from build123d import *

# Parameters (mm, degrees)
F1_DEPTH = 63.5
F2_DEPTH = 63.5


with BuildPart() as f1:
    # F0 (on Top) → F1 (new body)
    with BuildSketch(Plane.XY):
        Polygon((61.167741, 31.75), (-65.832259, 31.75), (-65.58761, 0), (-2.332259, 0), (-2.332259, 12.7), (15.4492, 12.7), (61.167741, 12.7), align=None)
    extrude(amount=F1_DEPTH)

    # F0 (on Top) → F2 (join)
    with BuildSketch(Plane.XY):
        Polygon((61.167741, 31.75), (-65.832259, 31.75), (-65.58761, 0), (-2.332259, 0), (-2.332259, 12.7), (15.4492, 12.7), (61.167741, 12.7), align=None)
    extrude(amount=F2_DEPTH)


solid = f1.part
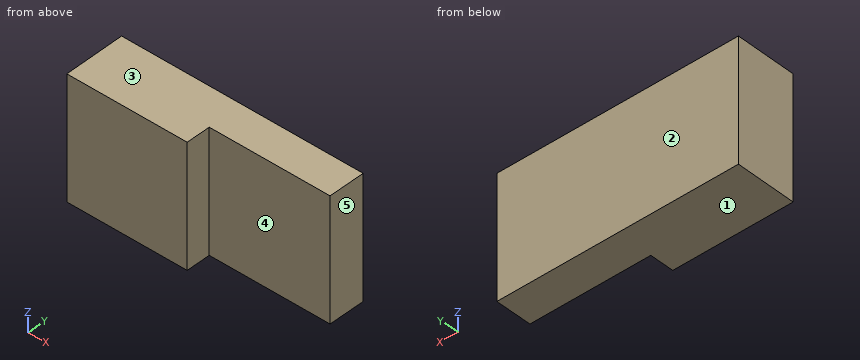
CAD build for the part. Positions are in the model's coordinates, mm. Face numbers are marked on the shaded views. A direction names the side the tool comes from. Coordinates: 2 decimals unless noted, no trailing zeros. Loops run counter-clockwise (first coordinate to the right, second up) from the corner with the lowest first, then second, coordinate; pieces in that order, holes last. Notation, with made-up numbers: (42, 78) - (46, 78) arc R20 cw to (46, 102) - close; hole circle Ø4 at (55, -21.5). An arc over 180 degrees is marked (long way). Use one line per item in the form item = value. Start each with the question number.
1) Band-saw the part on C-C (y = 6.5). Give the cut face in (x, z), and give its area (3 significant figures).
2) Tool access for the marked faces 4 and 5: list every direction of +Z, -Z, +X, -X, +Y, -Y with a clear straight run to the whole face (end or side of a thin tool).
3) Drill centre lines: L1, parallel to X at y = 29.5, z = 31; L2, parallel to X at y = 3, z = 21; L3, parallel to Y at x = 38.5, z = 41. Where is each one in solid material? Low to high. Write a range as from..to.
4) Two-plate mould, pull along Z, no slides. Class the marked faces 1, 2 and 3: +Z half, -Z half, draft (parallel to the pull), parting line (faces both ways), or undercut.
5) Band-saw the part on B-B (z = 5.5). Give the cut face in (x, y), and give its area (3 significant figures).
6) Band-saw the part on A-A (x = 13). Give the cut face in (y, z), and give its area (3 significant figures).
7) Flat gauge pin, fed straight in: pin 1 (10 mm diameter, centred on x = 26.5, z = 44, fed in from -Y). Where does the tip first touch, or does it go through?
Check values:
q1.outline = (-65.64, 0) - (-2.33, 0) - (-2.33, 63.5) - (-65.64, 63.5) - close
q1.area = 4,020 mm2
q2.face_4 = +Z, -Z, +X, -Y
q2.face_5 = +Z, -Z, +X, +Y, -Y
q3.L1 = -65.81..61.17
q3.L2 = -65.61..-2.33
q3.L3 = 12.7..31.75
q4.face_1 = -Z half
q4.face_2 = draft
q4.face_3 = +Z half
q5.outline = (-65.83, 31.75) - (-65.59, 0) - (-2.33, 0) - (-2.33, 12.7) - (61.17, 12.7) - (61.17, 31.75) - close
q5.area = 3,220 mm2
q6.outline = (12.7, 0) - (31.75, 0) - (31.75, 63.5) - (12.7, 63.5) - close
q6.area = 1,210 mm2
q7.pin_1 = 12.7
